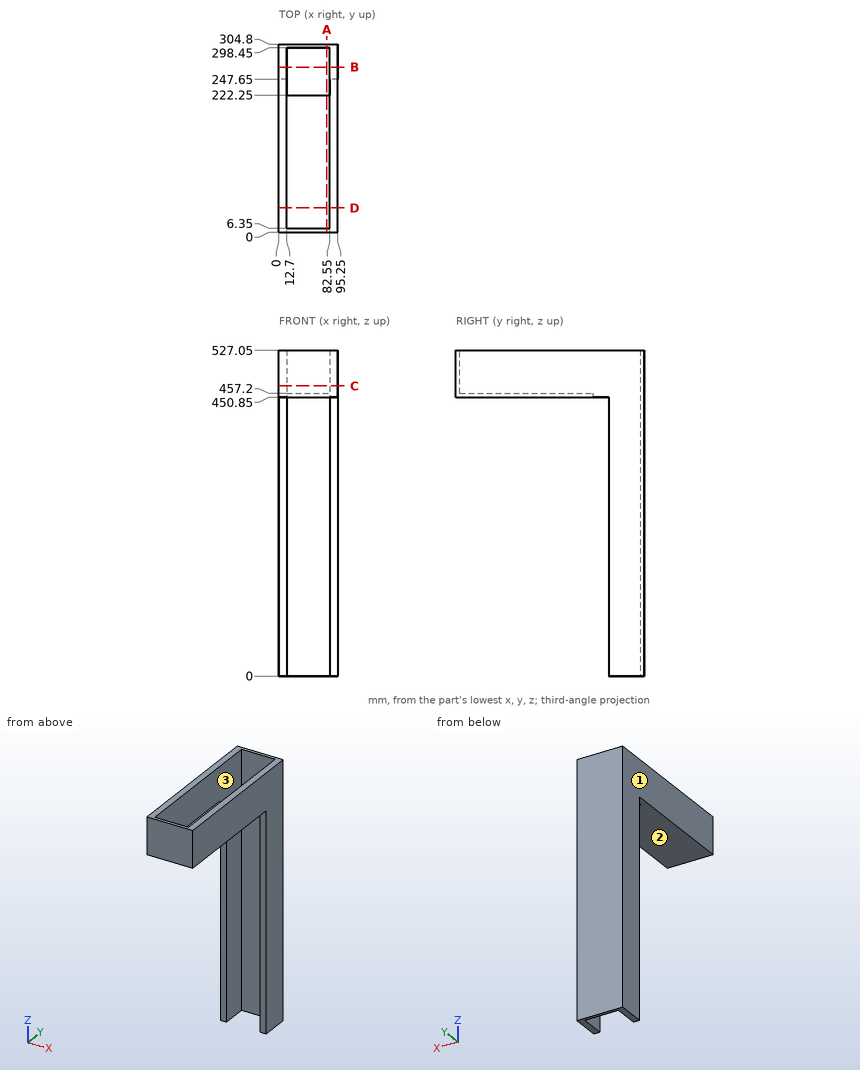
Geometry: see drawing. Coordinates: mm, zero at the bounding-box minimum. A direction names the side the tool comes from. Coordinates: 2 decimals unless noted, no trailing zeros. Loops run counter-clockwise (first coordinate to the right, second up) from the corner with the lowest first, then second, coordinate; pieces in that order, holes last. Notation, with made-up numbers: M 16,37.5 L 63,37.5 A20 ccw 63,62.5 Z; hole C 76.25,-8.75 d5. An arc over 180 degrees is marked long. Put each result on its own line as item: value. Start each with the question number.
1) Reachability of the marked faces 1, 2 and 3 from +Z, -Z, +X, -X, +Y, -Y: full face, straight path, thin tool, end or side. Return the list, or none.
2) Ray query, L1, parallel to Y at x = 33.5, z = 452.5; L2, parallel to X at y = 270.5, z = 58; L3, parallel to Z at x = 73, y = 140.5. Return the intervals inside material, ascending. Write a range as from..to.
3) Cut plane A-A on x = 77.5. Return the cut outline in (y, z).
4) Contact query for flat-ended pins moving along their axis: pin 1 Ø10 at (x, z) = (89.5, 241) entering from -Y; pin 2 Ø2 at (x, z) = (45, 398) entering from -Y; pin 3 Ø1 at (x, y) = (71, 101) entering from +Z. Output: stop coordinate, or through.
5) Cut plane B-B on y = 267.5. Return the cut outline in (x, z).
6) Cut plane C-C on z = 469.5. Return the cut outline in (x, y).
7) Cut plane D-D on y = 39.5. Return the cut outline in (x, z), then the cut area to 3 significant figures.
The answers:
1. face 1: +Z, -Z, -X, +Y, -Y
1. face 2: -Z, +X, -X, -Y
1. face 3: +Z
2. L1: y = 0..222.25, 298.45..304.8
2. L2: x = 0..12.7, 82.55..95.25
2. L3: z = 450.85..457.2
3. outline: M 0,450.85 L 222.25,450.85 L 222.25,457.2 L 6.35,457.2 L 6.35,527.05 L 0,527.05 Z; M 298.45,0 L 304.8,0 L 304.8,527.05 L 298.45,527.05 Z
4. pin 1: stops at y = 247.65
4. pin 2: stops at y = 298.45
4. pin 3: stops at z = 457.2
5. outline: M 0,0 L 12.7,0 L 12.7,527.05 L 0,527.05 Z; M 82.55,0 L 95.25,0 L 95.25,527.05 L 82.55,527.05 Z
6. outline: M 0,0 L 95.25,0 L 95.25,304.8 L 0,304.8 Z; hole M 12.7,6.35 L 82.55,6.35 L 82.55,298.45 L 12.7,298.45 Z
7. outline: M 0,450.85 L 95.25,450.85 L 95.25,527.05 L 82.55,527.05 L 82.55,457.2 L 12.7,457.2 L 12.7,527.05 L 0,527.05 Z
7. area: 2,380 mm²
